```python
from build123d import *

# Parameters (mm, degrees)
SKETCH1_W           = 65
SKETCH1_H           = 10
SKETCH1_R           = 1.5
BOSS_EXTRUDE1_DEPTH = 4.5
SKETCH2_W           = 58
SKETCH2_H           = 10
CUT_EXTRUDE1_DEPTH  = 1.75


with BuildPart() as part:
    # Sketch1 → Boss-Extrude1 (new body)
    with BuildSketch(Plane(origin=(0, 0, 0), x_dir=(1, 0, 0), z_dir=(0, 1, 0))):
        with Locations((32.5, 5)):
            Rectangle(SKETCH1_W, SKETCH1_H)
        with Locations(Location((13.75, 5, 0), (0, 0, 270))):
            Circle(SKETCH1_R, mode=Mode.SUBTRACT)
        with Locations(Location((32.5, 5, 0), (0, 0, 270))):
            Circle(SKETCH1_R, mode=Mode.SUBTRACT)
        with Locations(Location((51.25, 5, 0), (0, 0, 270))):
            Circle(SKETCH1_R, mode=Mode.SUBTRACT)
    extrude(amount=BOSS_EXTRUDE1_DEPTH)

    # Sketch2 → Cut-Extrude1 (cut)
    with BuildSketch(Plane.XZ):
        with Locations((32.5, -5)):
            Rectangle(SKETCH2_W, SKETCH2_H)
    extrude(amount=-CUT_EXTRUDE1_DEPTH, mode=Mode.SUBTRACT)


solid = part.part
```
Here's how the part is built. I have some questions about the finished solid (model axes, mm). A direction names the side the tool comes from. Coordinates: 2 decimals unless noted, no trailing zeros. Loops run counter-clockwise (first coordinate to the right, second up) from the corner with the lowest first, then second, coordinate; pieces in that order, holes last. Notation, with made-up numbers: (88.5, 28.5) - (99.5, 28.5) arc R10 cw to (99.5, 37.5) - close; hole circle Ø2 at (21, -26.75). An arc over 180 degrees is marked (long way). Answer as CSV lines item,"result".
Q1. If we section it at B-B, the plane x = 32.5: Write out the boundary of the cut face in (y, z), and give its area (4 significant figures).
Response:
outline,"(1.75, -10) - (4.5, -10) - (4.5, -6.5) - (1.75, -6.5) - close; (1.75, -3.5) - (4.5, -3.5) - (4.5, 0) - (1.75, 0) - close"
area,"19.25 mm2"
Q2. For faces 4 (the face through (31, 3, -5)), 5 (the face through (3.5, 1, -5)), which set-ups out of +Z, -Z, +X, -X, +Y, -Y let a thin tool reach every point of the face, with its end or its side?
Response:
face 4,"+Y, -Y"
face 5,"+Z, -Z, -Y"
Q3. If we section it at D-D, the plane x = 9.5: Write out the boundary of the cut face in (y, z), and give its area (3 significant figures).
Response:
outline,"(1.75, -10) - (4.5, -10) - (4.5, 0) - (1.75, 0) - close"
area,"27.5 mm2"
Q4. If I drill on L1, parallel to X at y = 2.7, z = -5; L2, parallel to X at y = 0.45, z = -4; L3, parallel to Z at x = 13.75, y = 2.95, over which ranges is the centre line in solid material (lowest first)? Write a range as [from, to].
Response:
L1,"[0, 12.25], [15.25, 31], [34, 49.75], [52.75, 65]"
L2,"[0, 3.5], [61.5, 65]"
L3,"[-10, -6.5], [-3.5, 0]"
Q5. We'd pull the mould along Z, two halves only. Please class faces 1 (the face through (32, 1.75, -3)), 2 (the face through (49.786, 3.106, -5.325)), 3 (the face through (32, 3, 0)): pulls with the +Z half, pulls with the -Z half, needs draft (parallel to the pull), parting line crosses it, or undercut.
Response:
face 1,"needs draft"
face 2,"undercut"
face 3,"pulls with the +Z half"
Q6. If we section it at A-A, the plane z = -5: Write out the boundary of the cut face in (x, y).
Response:
outline,"(0, 0) - (3.5, 0) - (3.5, 1.75) - (12.25, 1.75) - (12.25, 4.5) - (0, 4.5) - close; (15.25, 1.75) - (31, 1.75) - (31, 4.5) - (15.25, 4.5) - close; (34, 1.75) - (49.75, 1.75) - (49.75, 4.5) - (34, 4.5) - close; (52.75, 1.75) - (61.5, 1.75) - (61.5, 0) - (65, 0) - (65, 4.5) - (52.75, 4.5) - close"
Q7. For pin 1 (3.5 mm diameter, centred on x = 51.25, z = -5, fed in from -Y); pin 2 (1.9 mm diameter, centred on y = 0.5, z = -7, fed in from -X), each with a flat end and sliding along its axis, tell me the tip position at first contact or that it passes through.
Response:
pin 1,"y = 1.75"
pin 2,"x = 0"
Q8. If we section it at C-C, the plane z = -8.5: Write out the boundary of the cut face in (x, y), and give its area (3 significant figures).
Response:
outline,"(0, 0) - (3.5, 0) - (3.5, 1.75) - (61.5, 1.75) - (61.5, 0) - (65, 0) - (65, 4.5) - (0, 4.5) - close"
area,"191 mm2"
